Here's how the part is built. I have some questions about the finished solid (model axes, mm). A direction names the side the tool comes from. Give positions to 0.01 mm unless a question says otherwise; leave off trailing zeros. Write each loop counter-clockwise with the first axis right and the second up, starting at its lowest first coordinate (ties: lowest second). Pieces come first, ordered by that corner, then holes. Notation, with made-up numbers: (54, 66.25) -> (65, 66.25) arc R27 ccw to (65, 97.25) -> close; hole circle Ø7 at (13, -36.75). An arc over 180 degrees is marked (long way). Use one line per item in the form item = value.
Autodesk Inventor part; units mm, degrees
ref_plane "YZ Plane" through (0, 0, 0) normal (1, 0, 0) x (0, 1, 0)
ref_plane "XZ Plane" through (0, 0, 0) normal (0, 1, 0) x (-1, 0, 0)
ref_plane "XY Plane" through (0, 0, 0) normal (0, 0, 1) x (1, 0, 0)
sketch "Sketch1" plane through (0, 0, 0) normal (0, 0, 1) x (1, 0, 0)
  line L0 (0, 0) -> (116, 0)
  line L1 (116, 0) -> (116, 50)
  line L2 (116, 50) -> (0, 50)
  line L3 (0, 50) -> (0, 0)
  line L4 (0, 50) -> (3, 50)
  line L5 (3, 50) -> (3, 46.5)
  line L6 (3, 46.5) -> (0, 46.5)
  line L7 (0, 46.5) -> (0, 50)
  line L8 (0, 0) -> (3, 0)
  line L9 (3, 0) -> (3, 3.5)
  line L10 (3, 3.5) -> (0, 3.5)
  line L11 (0, 3.5) -> (0, 0)
  line L12 (58, 0) -> (58, 50) construction
  line L13 (113, 50) -> (113, 46.5)
  line L14 (113, 46.5) -> (116, 46.5)
  line L15 (113, 0) -> (113, 3.5)
  line L16 (113, 3.5) -> (116, 3.5)
  line L17 (19.5, 46.5) -> (96.5, 46.5) construction
  line L18 (96.5, 46.5) -> (96.5, 3.5) construction
  line L19 (96.5, 3.5) -> (19.5, 3.5) construction
  line L20 (19.5, 3.5) -> (19.5, 46.5) construction
  line L21 (28.5, 46.5) -> (89.5, 46.5)
  line L22 (89.5, 46.5) -> (89.5, 3.5)
  line L23 (89.5, 3.5) -> (28.5, 3.5)
  line L24 (28.5, 3.5) -> (28.5, 46.5)
  point P0 (1.5, 25)
  point P1 (0, 25)
  point P2 (1.5, 3.5)
  point P3 (19.5, 25)
  point P4 (58, 46.5)
  point P5 (1.5, 46.5)
  point P6 (94.5, 5.5)
  point P7 (94.5, 44.5)
  point P8 (26, 44.5)
  point P9 (26, 5.5)
  point P10 (0, 46.5)
  point P11 (0, 3.5)
  dimension "d0" = 116
  dimension "d1" = 50
  dimension "d2" = 3
  dimension "d4" = 21.5
  dimension "d5" = 21.5
  dimension "d6" = 77
  dimension "d7" = 61
  dimension "d8" = 9
  dimension "d9" = 2
  dimension "d10" = 2
  dimension "d11" = 2
  dimension "d12" = 6.5
  dimension "d13" = 2
extrude "Extrusion1" add sketch "Sketch1" along normal blind 3 contours L9 L10 L3 L6 L5 L2 L13 L14 L1 L16 L15 L0
sketch "Sketch2" plane through (0, 0, 3) normal (0, 0, 1) x (1, 0, 0)
  line L0 (28.5, 46.5) -> (89.5, 46.5)
  line L1 (19.5, 46.5) -> (96.5, 46.5)
  line L2 (96.5, 46.5) -> (96.5, 3.5)
  line L3 (96.5, 3.5) -> (19.5, 3.5)
  line L4 (19.5, 3.5) -> (19.5, 46.5)
  line L5 (113, 50) -> (3, 50)
  line L6 (0, 46.5) -> (0, 3.5)
  point P0 (0, 0)
  point P1 (26.42, 43.5)
  point P2 (26.42, 6.5)
  point P3 (58, 46.5)
  point P4 (58, 50)
  point P5 (19.5, 25)
  point P6 (0, 25)
  point P7 (93.5, 43.5)
  point P8 (93.5, 6.5)
  dimension "d17" = 77
  dimension "d18" = 3
  dimension "d19" = 3
  dimension "d20" = 3
  dimension "d28" = 6.92
hole "Hole1" at (26.42, 43.5, 3) at (26.42, 6.5, 3) at (93.5, 6.5, 3) at (93.5, 43.5, 3) direction (0, 0, -1) diameter 3 end through all
properties part number "pantallaSoport"
Q1. Will these pins go through, and if not, where does the flat tip stop? pin 1 Ø12 at (x, y) = (21.5, 13.5) entering from -Z; pin 2 Ø1.5 at (y, z) = (2, 1.5) entering from +X; pin 3 Ø1.5 at (y, z) = (47.5, 1.5) entering from -X; pin 4 Ø0.9 at (x, z) = (2, 2) entering from -Y.
Result set:
pin_1 = 0
pin_2 = 113
pin_3 = 3
pin_4 = 3.5
Q2. I want a section at B-B, the plane x = 72.5. Write out the boundary of the cut face in (y, z).
Result set:
outline = (0, 0) -> (3.5, 0) -> (3.5, 3) -> (0, 3) -> close; (46.5, 0) -> (50, 0) -> (50, 3) -> (46.5, 3) -> close
Q3. If we mould it in two halves opening along X, with no side actions, what happens to faces 1 (the face through (57, 0, 1)), 2 (the face through (113, 48, 1)), 3 (the face through (59, 46.5, 1)), 4 (the face through (59, 3.5, 1))? For each: +X half, -X half, draft (parallel to the pull), parting line (faces both ways), or undercut.
Result set:
face_1 = draft
face_2 = +X half
face_3 = undercut
face_4 = undercut
Q4. If I drill on line 1 along X through (y, z) = (6.5, 1.45); line 2 along Y through (x, z) = (26.42, 0.85); line 3 along Y through (x, z) = (75, 0.4), over which ranges is the centre line in solid material (lowest first)? Write a range as from..to.
Result set:
line_1 = 0..24.92, 27.92..28.5, 89.5..92, 95..116
line_2 = 0..5, 8..42, 45..50
line_3 = 0..3.5, 46.5..50
Q5. I want a section at A-A, the plane y = 6.5. Write out the boundary of the cut face in (x, z), and give its area (3 significant figures).
Result set:
outline = (0, 0) -> (24.92, 0) -> (24.92, 3) -> (0, 3) -> close; (27.92, 0) -> (28.5, 0) -> (28.5, 3) -> (27.92, 3) -> close; (89.5, 0) -> (92, 0) -> (92, 3) -> (89.5, 3) -> close; (95, 0) -> (116, 0) -> (116, 3) -> (95, 3) -> close
area = 147 mm2
Q6. I want a section at D-D, the plane z = 2.35. Write out the boundary of the cut face in (x, y).
Result set:
outline = (0, 3.5) -> (3, 3.5) -> (3, 0) -> (113, 0) -> (113, 3.5) -> (116, 3.5) -> (116, 46.5) -> (113, 46.5) -> (113, 50) -> (3, 50) -> (3, 46.5) -> (0, 46.5) -> close; hole circle Ø3 at (26.42, 6.5); hole circle Ø3 at (26.42, 43.5); hole (28.5, 3.5) -> (89.5, 3.5) -> (89.5, 46.5) -> (28.5, 46.5) -> close; hole circle Ø3 at (93.5, 6.5); hole circle Ø3 at (93.5, 43.5)
Q7. I want a section at C-C, the plane x = 93.5. Write out the boundary of the cut face in (y, z).
Result set:
outline = (0, 0) -> (5, 0) -> (5, 3) -> (0, 3) -> close; (8, 0) -> (42, 0) -> (42, 3) -> (8, 3) -> close; (45, 0) -> (50, 0) -> (50, 3) -> (45, 3) -> close
Q8. Which directions (+Z, -Z, +X, -X, +Y, -Y) give clear straight access to the entire face, cutting with the end or side of a thin tool? Please do faces 5 (the face through (114, 3.5, 1)), 6 (the face through (114, 46.5, 1)), 7 (the face through (89.5, 25, 1)), 8 (the face through (2, 46.5, 1)).
Result set:
face_5 = +Z, -Z, +X, -Y
face_6 = +Z, -Z, +X, +Y
face_7 = +Z, -Z
face_8 = +Z, -Z, -X, +Y
